Autodesk Inventor part; units mm, degrees
ref_plane "YZ Plane" through (0, 0, 0) normal (1, 0, 0) x (0, 1, 0)
ref_plane "XZ Plane" through (0, 0, 0) normal (0, 1, 0) x (-1, 0, 0)
ref_plane "XY Plane" through (0, 0, 0) normal (0, 0, 1) x (1, 0, 0)
sketch "Sketch1" plane through (0, 0, 0) normal (0, 1, 0) x (-1, 0, 0)
  line L0 (20, 10) -> (-20, 10)
  line L1 (-20, 10) -> (-20, -10)
  line L2 (-20, -10) -> (20, -10)
  line L3 (20, -10) -> (20, 10)
  line L4 (20, 10) -> (-20, -10) construction
  line L5 (-20, 10) -> (20, -10) construction
  line L6 (-30, 20) -> (30, 20)
  line L7 (30, 20) -> (30, -20)
  line L8 (30, -20) -> (-30, -20)
  line L9 (-30, -20) -> (-30, 20)
  line L10 (30, 0) -> (-30, 0) construction
  line L11 (-20, 0) -> (-10, 0) construction
  line L12 (-10, 10) -> (-10, -10) construction
  line L13 (20, 10) -> (10, 10) construction
  line L14 (10, 10) -> (10, -10) construction
  point P0 (0, 0)
  dimension "d0" = 40
  dimension "d1" = 20
  dimension "d2" = 10
  dimension "d3" = 10
  dimension "d4" = 10
extrude "Extrusion1" add sketch "Sketch1" along normal blind 80
sketch "Sketch2" plane through (-30, 0, 20) normal (0, 0, 1) x (1, 0, 0)
  line L0 (0, 0) -> (0, 80)
  line L1 (0, 40) -> (20, 40) construction
  line L2 (60, 0) -> (60, 80)
  line L3 (60, 40) -> (40, 40) construction
  line L4 (50, 0) -> (10, 0)
  line L5 (20, 0) -> (20, 70) construction
  line L6 (40, 0) -> (40, 80) construction
  line L7 (60, 80) -> (0, 80)
  line L8 (20, 65) -> (20, 15) construction
  line L9 (15.1, 65) -> (15.1, 15)
  line L10 (24.9, 15) -> (24.9, 65)
  arc A0 (24.9, 65) -> (15.1, 65) centre (20, 65) ccw
  arc A1 (15.1, 15) -> (24.9, 15) centre (20, 15) ccw
  line L11 (40, 65) -> (40, 15) construction
  line L12 (35.1, 65) -> (35.1, 15)
  line L13 (44.9, 15) -> (44.9, 65)
  arc A2 (44.9, 65) -> (35.1, 65) centre (40, 65) ccw
  arc A3 (35.1, 15) -> (44.9, 15) centre (40, 15) ccw
  point P0 (30, 0)
  dimension "d7" = 20
  dimension "d8" = 20
  dimension "d9" = 25
  dimension "d10" = 9.8
  dimension "d11" = 9.8
extrude "Extrusion2" cut sketch "Sketch2" against normal through all
sketch "Sketch3" plane through (-30, 0, -20) normal (-1, 0, 0) x (0, 0, 1)
  line L0 (20, 0) -> (20, 79.4763) construction
  line L1 (20, 64.7382) -> (20, 14.7382) construction
  line L2 (15.1, 64.7382) -> (15.1, 14.7382)
  line L3 (24.9, 14.7382) -> (24.9, 64.7382)
  arc A0 (24.9, 64.7382) -> (15.1, 64.7382) centre (20, 64.7382) ccw
  arc A1 (15.1, 14.7382) -> (24.9, 14.7382) centre (20, 14.7382) ccw
  point P0 (20, 39.7382)
  dimension "d14" = 25
  dimension "d15" = 9.8
extrude "Extrusion3" cut sketch "Sketch3" against normal blind 10
sketch "Sketch5" plane through (0, 80, 0) normal (0, 1, 0) x (1, 0, 0)
  line L0 (-20, 10) -> (20, 10)
  line L1 (30, -20) -> (30, 20)
  line L2 (20, 10) -> (30, 10)
  line L3 (30, 10) -> (30, -10)
  line L4 (30, -10) -> (20, -10)
  line L5 (20, -10) -> (20, 10)
  point P0 (0, 0)
  dimension "d18" = 20
extrude "Extrusion4" cut sketch "Sketch5" against normal through all
fillet "Fillet1" radius 4.25 4 edges at (30, 40, 10) (30, 40, -10) (30, 40, -20) (30, 40, 20)
fillet "Fillet2" radius 4.75 2 edges at (-30, 40, 20) (-30, 40, -20)
properties part number "VerticalBeamMount" material "ABS Plastic"
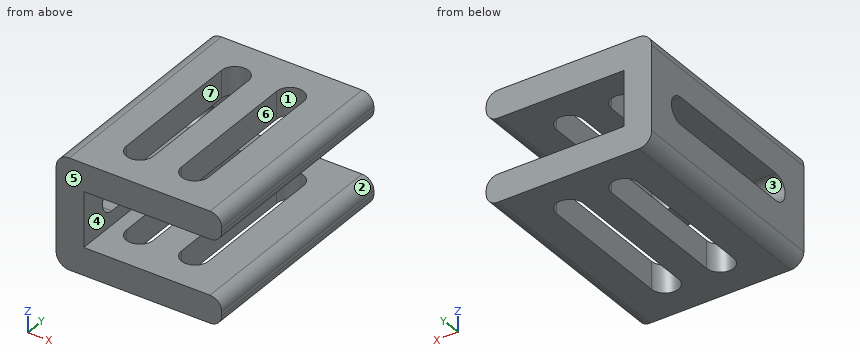
Work out the finished part from the listing and answer in its coordinate system (mm). Face numbers are marked on the shaded views. A direction names the side the tool comes from. Coordinates: 2 decimals unless noted, no trailing zeros. Write each loop counter-clockwise with the first axis right and the second up, starting at its lowest first coordinate (ties: lowest second). Pieces come first, ordered by that corner, then holes. Notation, with made-up numbers: (4, 47) - (34, 47) arc R20 cw to (34, 59) - close; hole circle Ø4 at (25, 35.5). An arc over 180 degrees is marked (long way). One line per question, with ' | ' between items.
1) Find section A-A, the plane x = 2.5. Determine the outline of the cut face in (y, z).
Checks:
outline: (0, -20) - (80, -20) - (80, -10) - (0, -10) - close; (0, 10) - (80, 10) - (80, 20) - (0, 20) - close
2) Find section B-B, the plane y = 63. Give the number of separate pieces and of enclosed holes in the cut face, and give its area (3 significant figures).
Checks:
separate pieces: 6 | enclosed holes: 0 | area: 885 mm2
3) Flat-ended cylindrical pins translate along their axes: P1, Ø3, axis at x = -13, z = -7, coming from the -Y side; P2, Ø22, axis at y = 30.5, z = 3, coming from the +X side. Find the tip coordinate at first contact, or state that the pin passes through.
Checks:
P1: through | P2: x = 29.99
4) Find section C-C, the plane x = -10. Determine the outline of the cut face in (y, z), and give its area (3 significant figures).
Checks:
outline: (0, -20) - (10.1, -20) - (10.1, -10) - (0, -10) - close; (0, 10) - (10.1, 10) - (10.1, 20) - (0, 20) - close; (69.9, -20) - (80, -20) - (80, -10) - (69.9, -10) - close; (69.9, 10) - (80, 10) - (80, 20) - (69.9, 20) - close | area: 404 mm2
5) Find section D-D, the plane z = 0. Determine the outline of the cut face in (x, y), and give its area (3 significant figures).
Checks:
outline: (-30, 0) - (-20, 0) - (-20, 9.84) - (-30, 9.84) - close; (-30, 69.64) - (-20, 69.64) - (-20, 80) - (-30, 80) - close | area: 202 mm2
6) Consider probe 1 along X at (y, z) = (48.5, 15.5); probe 2 along Z at (x, y) = (7.5, 4); probe 3 along X at (y, z) = (66.5, 12.5). Determine where each line is inside the solid, lowest interval first. Write a range as [from, to].
Checks:
probe 1: [-29.99, -14.9], [-5.1, 5.1], [14.9, 30] | probe 2: [-20, -10], [10, 20] | probe 3: [-30, -14.66], [-5.34, 5.34], [14.66, 29.62]
7) For the marked faces 1, 2 and 3, determine the directions among +Z, -Z, +X, -X, +Y, -Y from which every point of the face is accessible in a straight line to the end or side of a thin tool.
Checks:
face 1: +Z, -Z | face 2: +X, +Y, -Y | face 3: +X, -X
8) The mould has two halves that part along X. Classify the marked faces 4, 5, 6 and 7: +X half, -X half, draft (parallel to the pull), parting line (faces both ways), or undercut.
Checks:
face 4: +X half | face 5: draft | face 6: undercut | face 7: undercut
